Autodesk Inventor part; units mm, degrees
ref_plane "YZ Plane" through (0, 0, 0) normal (1, 0, 0) x (0, 1, 0)
ref_plane "XZ Plane" through (0, 0, 0) normal (0, 1, 0) x (-1, 0, 0)
ref_plane "XY Plane" through (0, 0, 0) normal (0, 0, 1) x (1, 0, 0)
sketch "Sketch1" plane through (0, 0, 0) normal (0, 0, 1) x (1, 0, 0)
  line L0 (18.2242, 0) -> (206.7758, 0)
  line L1 (-6.65, 150) -> (231.65, 150)
  line L2 (-6.65, 150) -> (-0.8071, 18.2063)
  line L3 (225.8071, 18.2063) -> (231.65, 150)
  arc A0 (-0.8071, 18.2063) -> (18.2242, 0) centre (18.2242, 19.05) ccw
  arc A1 (206.7758, 0) -> (225.8071, 18.2063) centre (206.7758, 19.05) ccw
  line L4 (-14.1495, 62.3) -> (284.7503, 62.3)
  point P0 (0, 0)
  point P1 (225, 0)
  point P2 (112.5, 0)
  point P3 (112.5, 150)
  point P4 (227.762, 62.3)
  point P5 (-2.762, 62.3)
  dimension "d0" = 225
  dimension "d1" = 150
  dimension "d2" = 238.3
  dimension "d4" = 19.05
  dimension "d11" = 0
  dimension "d12" = 62.3
extrude "Extrusion1" add sketch "Sketch1" along normal blind 25.4 contours A0 L2 L4 L3 A1 L0
sketch "Sketch2" plane through (0, 0, 25.4) normal (0, 0, 1) x (1, 0, 0)
  line L0 (243.0343, 163.5066) -> (27.3006, 163.5066)
  line L1 (27.3006, 163.5066) -> (27.3006, 18.9917)
  line L2 (27.3006, 18.9917) -> (243.0343, 18.9917)
  line L3 (243.0343, 18.9917) -> (243.0343, 163.5066)
  line L4 (27.1522, 18.9917) -> (243.0343, 18.9917)
  line L5 (243.0343, 18.9917) -> (243.0343, -17.0628)
  line L6 (243.0343, -17.0628) -> (27.1522, -17.0628)
  line L7 (27.1522, -17.0628) -> (27.1522, 18.9917)
  point P0 (0, 0)
extrude "Test" [suppressed]
properties part number "Divider_3DPrint"
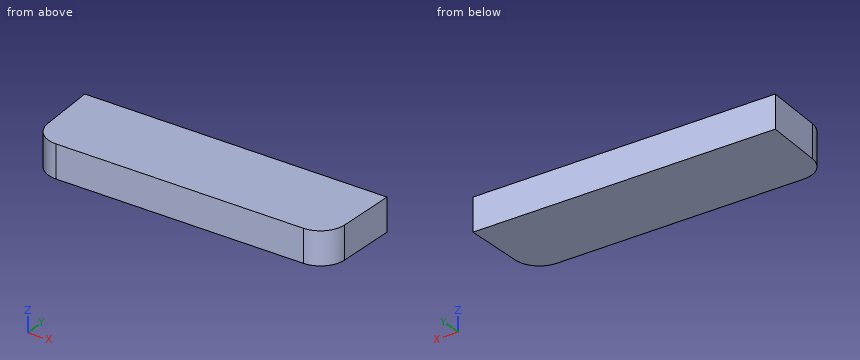
Geometry check sheet. Reference: the model listing, model coordinates, mm. Give positions to 0.01 mm unless a question says otherwise; leave off trailing zeros. Order: outer loops, then holes, each group sorted by start corner. A loop starts at its lowest first (then second) coordinate and runs counter-clockwise, first axis right, second up. Notation, with made-up numbers: (19, 64.5) - (54, 64.5) arc R16 ccw to (54, 89.5) - close; hole circle Ø4 at (26.25, 59). An arc over 180 degrees is marked (long way). Write item = value, one per line. Start each with the question number.
1) Section check A-A (z = 20.25). Enter the section's corners in (x, y).
2) Section check B-B (y = 11.5). Enter the section's corners in (x, z).
3) Scan lines: L1, parallel to X at y = 37, z = 13.75; L2, parallel to X at y = 33.5, z = 14.5; L3, parallel to Y at x = 218, z = 19.5. Record each from-to range of solid material in increasing order.
4) Gauge pin test, flat ends, axial feed: pin 1 Ø8 at (y, z) = (41.5, 4.5) entering from +X; pin 2 Ø4 at (y, z) = (7.5, 13.5) entering from -X; pin 3 Ø4 at (y, z) = (43.5, 15) entering from -X. Record the tip position at first contact, or that the pin passes through.
Geometry check:
q1.outline = (-2.76, 62.3) - (-0.81, 18.21) arc R19.05 ccw to (18.22, 0) - (206.78, 0) arc R19.05 ccw to (225.81, 18.21) - (227.76, 62.3) - close
q2.outline = (0.73, 0) - (224.27, 0) - (224.27, 25.4) - (0.73, 25.4) - close
q3.L1 = -1.64 to 226.64
q3.L2 = -1.49 to 226.49
q3.L3 = 3.66 to 62.3
q4.pin_1 = 227.02
q4.pin_2 = 1.74
q4.pin_3 = -2.02
